Autodesk Inventor part; units mm, degrees
ref_plane "YZ Plane" through (0, 0, 0) normal (1, 0, 0) x (0, 1, 0)
ref_plane "XZ Plane" through (0, 0, 0) normal (0, 1, 0) x (-1, 0, 0)
ref_plane "XY Plane" through (0, 0, 0) normal (0, 0, 1) x (1, 0, 0)
sketch "草圖1" plane through (0, 0, 0) normal (0, 1, 0) x (-1, 0, 0)
  line L0 (0, 0) -> (40, 0)
  line L1 (40, 0) -> (40, -10)
  line L2 (40, -10) -> (0, -10)
  line L3 (0, -10) -> (0, 0)
  line L4 (0, 0) -> (10, 0)
  line L5 (10, 0) -> (10, -10)
  line L6 (10, -10) -> (0, -10)
  line L7 (0, -10) -> (0, 0)
  line L8 (40, 0) -> (30, 0)
  line L9 (30, 0) -> (30, -10)
  line L10 (30, -10) -> (40, -10)
  line L11 (40, -10) -> (40, 0)
  circle A0 centre (7.5, -2.5) radius 1.7
  circle A1 centre (7.5, -7.5) radius 1.7
  circle A2 centre (2.5, -2.5) radius 1.7
  circle A3 centre (2.5, -7.5) radius 1.7
  line L12 (20, 0) -> (20, -10) construction
  circle A4 centre (32.5, -2.5) radius 1.7
  circle A5 centre (32.5, -7.5) radius 1.7
  circle A6 centre (37.5, -2.5) radius 1.7
  circle A7 centre (37.5, -7.5) radius 1.7
  dimension "d0" = 40
  dimension "d1" = 10
  dimension "d2" = 10
  dimension "d3" = 10
  dimension "d4" = 10
  dimension "d5" = 10
  dimension "d6" = 3.4
  dimension "d7" = 2.5
  dimension "d8" = 2.5
  dimension "d11" = 5
  dimension "d14" = 5
extrude "擠出1" add sketch "草圖1" along normal blind 5 contours L0 L5 L2 L3 | L0 L1 L2 L9 | A0 | A1 | A2 | A3 | A4 | A5 | A6 | A7
extrude "擠出2" cut sketch "草圖1" along normal blind 1.5 contours A0 | A1 | A2 | A3 | A4 | A5 | A6 | A7
sketch "草圖2" plane through (0, 0, 0) normal (0, 0, 1) x (1, 0, 0)
  line L0 (-40, 0) -> (-30, 0)
  line L1 (-30, 0) -> (-30, 5)
  line L2 (-40, 5) -> (-30, 5)
  line L3 (-40, 0) -> (-40, 5)
  line L4 (-10, 0) -> (0, 0)
  line L5 (0, 0) -> (0, 5)
  line L6 (-10, 5) -> (0, 5)
  line L7 (-10, 0) -> (-10, 5)
  line L8 (-30, 5) -> (-10, 5) construction
  line L9 (-10, 0) -> (-10, 5) construction
  arc A0 (-10, 5) -> (-30, 5) centre (-20, 5) ccw
  line L10 (-5.8579, 0) -> (-10, 0) construction
  arc A1 (-5, 5) -> (-35, 5) centre (-20, 5) ccw
  dimension "d21" = 5
extrude "擠出3" add sketch "草圖2" against normal blind 10 contours L2 A1 L6 A0
sketch "草圖3" plane through (0, 5, 0) normal (0, 1, 0) x (1, 0, 0)
  circle A0 centre (-2.5, 7.5) radius 1.7
  point P0 (0, 0)
extrude "擠出4" add sketch "草圖3" along normal blind 1.5
pattern_linear "矩形陣列1" count 2 spacing 5 along (0, 0, 1) count 2 spacing 35 along (-1, 0, 0) of "擠出4"
properties part number "110033226_ipt_40_背流拱橋"
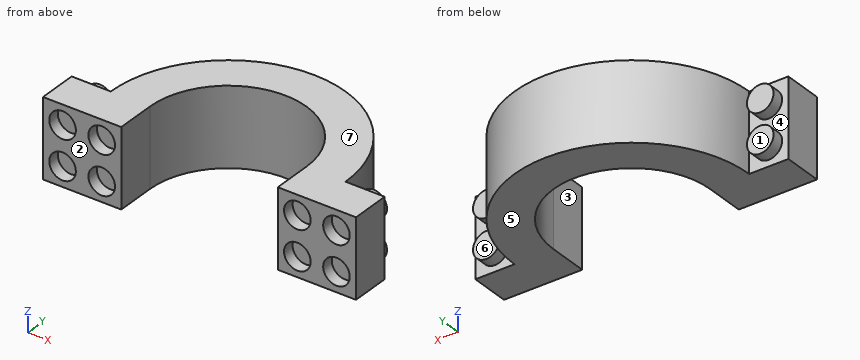
Source: CAD feature listing. Evaluate the final solid. Frame: model axes, mm. Face numbers are marked on the shaded views. A direction names the side the tool comes from. Round coordinates to 2 decimals unless told otherwise and drop trailing zeros. Loops run counter-clockwise (first coordinate to the right, second up) from the corner with the lowest first, then second, coordinate; pieces in that order, holes last.
(1) Access query for the marked faces 1, 2 and 3. Directions: +Z, -Z, +X, -X, +Y, -Y. A direction counts if a zero-diameter tool reaches every point of the face in a straight line with its end or side. Return the directions, or none.
From the geometry:
face 1: +Z, -Z, -X, +Y
face 2: +Z, -Z, +X, -X, -Y
face 3: +Z, -Z, -Y
(2) Section query C-C (x = -7.5). Output: boundary loops of the cut face in (y, z), and give its area (3 significant figures).
From the geometry:
outline: (0, -10) - (13.29, -10) - (13.29, 0) - (0, 0) - (0, -0.8) - (1.5, -0.8) - (1.5, -4.2) - (0, -4.2) - (0, -5.8) - (1.5, -5.8) - (1.5, -9.2) - (0, -9.2) - close
area: 123 mm2
(3) Pull-direction query (Z, two-part tool) for the marked faces 4, 5, 6 and 7; classes: +Z half, -Z half, draft (parallel to the pull), parting line (faces both ways), or undercut.
From the geometry:
face 4: undercut
face 5: -Z half
face 6: draft
face 7: +Z half
(4) Section query D-D (z = -5). Output: boundary loops of the cut face in (x, y), and give its area (3 significant figures).
From the geometry:
outline: (-40, 0) - (-30, 0) - (-30, 5) arc R10 cw to (-10, 5) - (-10, 0) - (0, 0) - (0, 5) - (-5, 5) arc R15 ccw to (-35, 5) - (-40, 5) - close
area: 296 mm2
(5) Section query B-B (y = 11.25). Output: boundary loops of the cut face in (x, z).
From the geometry:
outline: (-33.64, -10) - (-27.81, -10) - (-27.81, 0) - (-33.64, 0) - close; (-12.19, -10) - (-6.36, -10) - (-6.36, 0) - (-12.19, 0) - close
(6) Material intervals for probe 1 along Z at (x, y) = (-32.5, 0.85); probe 2 along X at (y, z) = (1.75, -9.25); probe 3 along X at (y, z) = (1.25, -2), sorted ascending.
From the geometry:
probe 1: z = -10 to -9.2, -5.8 to -4.2, -0.8 to 0
probe 2: x = -40 to -30, -10 to 0
probe 3: x = -40 to -39.12, -35.88 to -34.12, -30.88 to -30, -10 to -9.12, -5.88 to -4.12, -0.88 to 0
(7) Contact query for flat-ended pins moving along their axis: pin 1 Ø5.5 at (x, z) = (-2, -6) entering from +Y; pin 2 Ø1.5 at (x, z) = (-25, -7) entering from -Y; pin 3 Ø1.7 at (x, z) = (-2.5, -7) entering from -Y. Output: stop coordinate, or through.
From the geometry:
pin 1: stops at y = 6.5
pin 2: stops at y = 13.18
pin 3: stops at y = 1.5
